Can you work these out from the drawing? Everything is in mm from the part's minimum corner. Coordinates: 2 decimals unless noted, no trailing zeros. Loops run counter-clockwise (first coordinate to the right, second up) from the corner with the lowest first, then second, coordinate; pieces in that order, holes last.
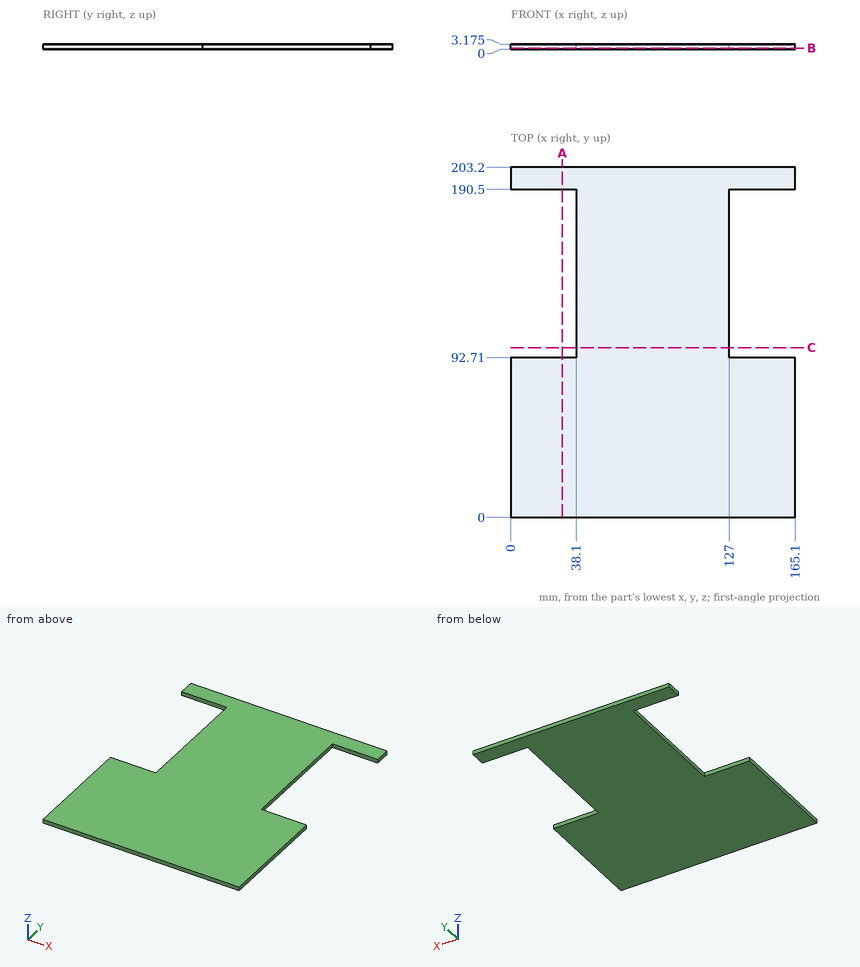
1) Imagine slicing it at A-A on x = 30. List the corners of the cut face in (y, z) for me (3 decimals), plus the area to 3 significant figures.
2) If I drill on L1, parallel to Y at x = 34, z = 1.05; L2, parallel to X at y = 186, z = 0.15, over which ranges is the centre line in solid material (lowest first)?
3) Will this pin go through, and if not, where does the flat tip stop? pin 1 (1 mm diameter, centred on y = 165, z = 2, fed in from +X).
4) Imagine slicing it at B-B on z = 0.8. List the corners of the cut face in (x, y) for me.
5) Imagine slicing it at C-C on y = 98.5. List the corners of the cut face in (x, z) for me (3 decimals), plus the area to 3 significant figures.
Solved:
1. outline: (0, 0) - (92.71, 0) - (92.71, 3.175) - (0, 3.175) - close; (190.5, 0) - (203.2, 0) - (203.2, 3.175) - (190.5, 3.175) - close
1. area: 335 mm2
2. L1: y = 0 to 92.71, 190.5 to 203.2
2. L2: x = 38.1 to 127
3. pin 1: stops at x = 127
4. outline: (0, 0) - (165.1, 0) - (165.1, 92.71) - (127, 92.71) - (127, 190.5) - (165.1, 190.5) - (165.1, 203.2) - (0, 203.2) - (0, 190.5) - (38.1, 190.5) - (38.1, 92.71) - (0, 92.71) - close
5. outline: (38.1, 0) - (127, 0) - (127, 3.175) - (38.1, 3.175) - close
5. area: 282 mm2
